Source: three-view drawing plus pictorial views. Frame: mm from the lowest corner of the part. A direction names the side the tool comes from. Give positions to 0.01 mm unless a question says otherwise; leave off trailing zeros. Order: outer loops, then holes, each group sorted by start corner. A loop starts at its lowest first (then second) coordinate and runs counter-clockwise, first axis right, second up. Notation, with made-up numbers: M -16,43 L 22,43 A28 cw 22,62 Z; hole C 17.5,30.25 d1. An arc over 180 degrees is marked long. One line per item, written item: value. Start each with the question number.
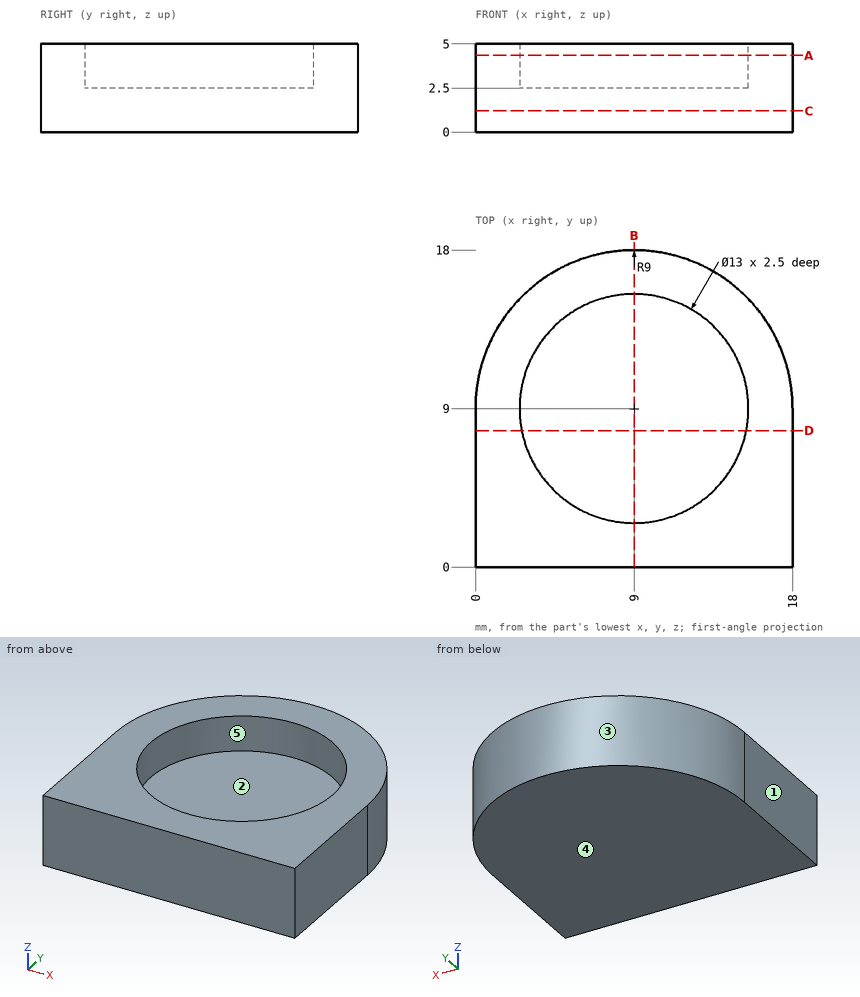
Q1. Ray query, line 1 along Y through (x, z) = (9, 4.45); line 2 along Z through (x, y) = (9, 9); line 3 along X through (y, z) = (3.25, 3.4). Return the intervals inside material, ascending. Write a range as [from, to].
Q2. Mould query, pull axis Y, two halves, no side actions, for the marked faces 1, 2 and 3. Classes: +Y half, -Y half, draft (parallel to the pull), parting line (faces both ways), or undercut.
Q3. Section query B-B on x = 9. Return loops of the section in (y, z), and give its area (3 significant figures).
Q4. Section query D-D on y = 7.75. Return loops of the section in (x, z).
Q5. Section query A-A on z = 4.35. Return loops of the section in (x, y).
Q6. Set-up query: the marked faces 4 and 5. Return all of +Z, -Z, +X, -X, +Y, -Y with unobstructed straight access to the full face (end or side cutting, diameter ignored); none if empty.
Q7. Section query C-C on z = 1.2. Return loops of the section in (x, y).
Q8. Contact query for flat-ended pins moving along their axis: pin 1 (1 mm diameter, centred on x = 10.5, y = 8.5, fed in from +Z); pin 2 (1 mm diameter, centred on x = 7, z = 1, fed in from +Y). Output: stop coordinate, or through.
Results below:
1. line 1: [0, 2.5], [15.5, 18]
1. line 2: [0, 2.5]
1. line 3: [0, 5.97], [12.03, 18]
2. face 1: draft
2. face 2: undercut
2. face 3: +Y half
3. outline: M 0,0 L 18,0 L 18,5 L 15.5,5 L 15.5,2.5 L 2.5,2.5 L 2.5,5 L 0,5 Z
3. area: 57.5 mm2
4. outline: M 0,0 L 18,0 L 18,5 L 15.38,5 L 15.38,2.5 L 2.62,2.5 L 2.62,5 L 0,5 Z
5. outline: M 0,0 L 18,0 L 18,9 A9 ccw 0,9 Z; hole C 9,9 d13
6. face 4: -Z, +X, -X, +Y, -Y
6. face 5: +Z
7. outline: M 0,0 L 18,0 L 18,9 A9 ccw 0,9 Z
8. pin 1: z = 2.5
8. pin 2: y = 17.87
